Here's how the part is built. I have some questions about the finished solid (model axes, mm). A direction names the side the tool comes from. Give positions to 0.01 mm unless a question says otherwise; leave off trailing zeros. Loops run counter-clockwise (first coordinate to the right, second up) from the corner with the lowest first, then second, coordinate; pieces in that order, holes last. Notation, with made-up numbers: (44, -25) - (94, -25) arc R17 cw to (94, -7) - close; hole circle Ø5 at (67, -33.75). An arc over 180 degrees is marked (long way). Return JSON: item names as keys, results as strings. Group by question number.
(1) I need wall thicknesses on probe 1 along X at (y, z) = (10.25, 7.5) (3 decimals); probe 2 along Z at (x, y) = (19, 5.5) (3 decimals); probe 3 along X at (y, z) = (10.5, -8.5) (3 decimals). Which ranges of each line are inside material? Lowest first, please. Write a range as [from, to].
(2) If we section it at B-B (x = -4): Please give me the cut outline in (y, z) (3 decimals).
(3) If we section it at C-C (z = 5): Please give me the cut outline in (x, y) (3 decimals).
(4) On a 3-axis mill with a long thin cutter (end or side, diameter ignored), from which of +Z, -Z, +X, -X, +Y, -Y can I reach the whole of each face in a straight line? I mean faces 3 (the cylindrical face through (24.81, 14.64, -4.33)), 4 (the flat face through (22.5, -0.6, -8.985)), 5 (the flat face through (-23.6, -0.6, 8.985)). Say none if no direction works.
(5) For P1, Ø10, axis at x = -11, z = 5.5, coming from the +Y side; P2, Ø5, axis at x = -19, z = 4.5, coming from the -Y side; P3, Ø4, axis at x = 13.475, z = -11.175, coming from the -Y side; P4, Ø1.8, axis at x = -13.495, z = -11.175, coming from the +Y side, each with a flat end and sliding along its axis, tell me the tip position at first contact or that it passes through.
(6) If we mould it in two halves opening along X, with no side actions, what happens to faces 1 (the flat face through (12, -1.12, -11)), 2 (the cylindrical face through (-14.685, 2.007, -10.262))? For each: released by +X, released by -X, zero draft, split by the parting line, or undercut.
(7) If we section it at A-A (y = 3.25): Please give me the cut outline in (x, z) (3 decimals), then the cut area to 3 significant figures.
```python
from build123d import *

# Parameters (mm, degrees)
SKETCH_1_W          = 54.61
SKETCH_1_H          = 29.97
EXTRUDE_1_DEPTH     = 2.5
EXTRUDE_2_DEPTH     = 17
CUT_EXTRUDE_1_DEPTH = 30.97
SKETCH_4_R          = 1.145
CUT_EXTRUDE_2_DEPTH = 3.5
SKETCH_5_R          = 2.25
SKETCH_5_W          = 7.5
SKETCH_5_H          = 6
SKETCH_5_W_2        = 9.5
EXTRUDE_3_DEPTH     = 1.12
SKETCH_6_R          = 1.145
CUT_EXTRUDE_3_DEPTH = 4.62
SKETCH_7_R          = 1.5
CUT_EXTRUDE_4_DEPTH = 1
SKETCH_9_W          = 0.66
SKETCH_9_H          = 0.76
EXTRUDE_5_DEPTH     = 3
SKETCH_10_R         = 3.75
EXTRUDE_6_DEPTH     = 1
SKETCH_11_R         = 3
SKETCH_11_R_2       = 2
EXTRUDE_7_DEPTH     = 4
SKETCH_12_R         = 4.25
SKETCH_12_R_2       = 3.25
EXTRUDE_8_DEPTH     = 4
SKETCH5_W           = 26
SKETCH5_H           = 4
CUT_EXTRUDE4_DEPTH  = 17
BOSS_EXTRUDE1_DEPTH = 18
SKETCH7_W           = 2
SKETCH7_H           = 29.97
BOSS_EXTRUDE2_DEPTH = 1


with BuildPart() as part:
    # Эскиз1 → Бобышка-Вытянуть1 (new body)
    with BuildSketch(Plane(origin=(0, 0, 0), x_dir=(1, 0, 0), z_dir=(0, 1, 0))):
        Rectangle(SKETCH_1_W, SKETCH_1_H)
    extrude(amount=EXTRUDE_1_DEPTH)

    # Эскиз2 → Бобышка-Вытянуть2 (add)
    with BuildSketch(Plane(origin=(0, 2.5, 0), x_dir=(1, 0, 0), z_dir=(0, 1, 0))):
        with BuildLine():
            Line((27.305, -14.985), (-0.695, -14.985))
            Line((-0.695, -14.985), (-0.695, -13.485))
            Line((-0.695, -13.485), (23.305, -13.485))
            ThreePointArc((23.305, -13.485), (24.719213562, -12.899213562), (25.305, -11.485))
            Line((25.305, -11.485), (25.305, 11.485))
            ThreePointArc((25.305, 11.485), (24.719213562, 12.899213562), (23.305, 13.485))
            Line((23.305, 13.485), (-0.695, 13.485))
            Line((-0.695, 13.485), (-0.695, 14.985))
            Line((-0.695, 14.985), (27.305, 14.985))
            Line((27.305, 14.985), (27.305, -14.985))
        make_face()
    extrude(amount=EXTRUDE_2_DEPTH)

    # Эскиз3 → Вырез-Вытянуть1 (cut, through all)
    with BuildSketch(Plane.XY.offset(14.985)):
        Polygon((-0.695, 2.5), (25.305, 19.5), (-0.695, 19.5), align=None)
    extrude(amount=-CUT_EXTRUDE_1_DEPTH, mode=Mode.SUBTRACT)

    # Эскиз4 → Вырез-Вытянуть2 (cut, through all)
    with BuildSketch(Plane(origin=(0, 2.5, 0), x_dir=(1, 0, 0), z_dir=(0, 1, 0))):
        with Locations((-13.495, 11.175)):
            Circle(SKETCH_4_R)
        with Locations((-0.005, -11.175)):
            Circle(SKETCH_4_R)
        with Locations((13.475, 11.175)):
            Circle(SKETCH_4_R)
    extrude(amount=-CUT_EXTRUDE_2_DEPTH, mode=Mode.SUBTRACT)

    # Эскиз5 → Бобышка-Вытянуть3 (add)
    with BuildSketch(Plane.XZ):
        with Locations((-0.005, 11.175)):
            Circle(SKETCH_5_R)
        with Locations((13.475, -11.175)):
            Circle(SKETCH_5_R)
        with Locations((-13.495, -11.175)):
            Circle(SKETCH_5_R)
        with Locations((-23.555, 11.985)):
            Rectangle(SKETCH_5_W, SKETCH_5_H)
        with Locations((22.555, 11.985)):
            Rectangle(SKETCH_5_W_2, SKETCH_5_H)
        with Locations((22.555, -11.985)):
            Rectangle(SKETCH_5_W_2, SKETCH_5_H)
        with Locations((-23.555, -11.985)):
            Rectangle(SKETCH_5_W, SKETCH_5_H)
    extrude(amount=EXTRUDE_3_DEPTH)

    # Эскиз6 → Вырез-Вытянуть3 (cut, through all)
    with BuildSketch(Plane(origin=(0, 2.5, 0), x_dir=(1, 0, 0), z_dir=(0, 1, 0))):
        with Locations((-13.495, 11.175)):
            Circle(SKETCH_6_R)
        with Locations((13.475, 11.175)):
            Circle(SKETCH_6_R)
        with Locations((-0.005, -11.175)):
            Circle(SKETCH_6_R)
    extrude(amount=-CUT_EXTRUDE_3_DEPTH, mode=Mode.SUBTRACT)

    # Эскиз7 → Вырез-Вытянуть4 (cut)
    with BuildSketch(Plane(origin=(0, 2.5, 0), x_dir=(1, 0, 0), z_dir=(0, 1, 0))):
        with Locations((-13.495, 11.175)):
            Circle(SKETCH_7_R)
        with Locations((13.475, 11.175)):
            Circle(SKETCH_7_R)
        with Locations((-0.005, -11.175)):
            Circle(SKETCH_7_R)
    extrude(amount=-CUT_EXTRUDE_4_DEPTH, mode=Mode.SUBTRACT)

    # Эскиз9 → Бобышка-Вытянуть5 (add)
    with BuildSketch(Plane.XZ):
        with Locations((25.075, 6.35)):
            Rectangle(SKETCH_9_W, SKETCH_9_H)
        with Locations((25.075, -6.35)):
            Rectangle(SKETCH_9_W, SKETCH_9_H)
    extrude(amount=EXTRUDE_5_DEPTH)

    # Эскиз10 → Бобышка-Вытянуть6 (add)
    with BuildSketch(Plane.ZY.offset(-25.305)):
        with Locations((-6.35, 11.48)):
            Circle(SKETCH_10_R)
        with Locations((6.35, 11.48)):
            Circle(SKETCH_10_R)
    extrude(amount=EXTRUDE_6_DEPTH)

    # Эскиз11 → Бобышка-Вытянуть7 (add)
    with BuildSketch(Plane.ZY.offset(-24.305)):
        with Locations((-6.35, 11.48)):
            Circle(SKETCH_11_R)
        with Locations((-6.35, 11.48)):
            Circle(SKETCH_11_R_2, mode=Mode.SUBTRACT)
    extrude(amount=EXTRUDE_7_DEPTH)

    # Эскиз12 → Бобышка-Вытянуть8 (add)
    with BuildSketch(Plane.ZY.offset(-24.305)):
        with Locations((6.35, 11.48)):
            Circle(SKETCH_12_R)
        with Locations((6.35, 11.48)):
            Circle(SKETCH_12_R_2, mode=Mode.SUBTRACT)
    extrude(amount=EXTRUDE_8_DEPTH)

    # Sketch5 → Cut-Extrude4 (cut)
    with BuildSketch(Plane(origin=(0, 19.5, 0), x_dir=(1, 0, 0), z_dir=(0, 1, 0))):
        with Locations((12.305, -12.985)):
            Rectangle(SKETCH5_W, SKETCH5_H)
        with Locations((12.305, 12.985)):
            Rectangle(SKETCH5_W, SKETCH5_H)
    extrude(amount=-CUT_EXTRUDE4_DEPTH, mode=Mode.SUBTRACT)

    # Sketch6 → Boss-Extrude1 (add)
    with BuildSketch(Plane(origin=(0, 2.5, 0), x_dir=(1, 0, 0), z_dir=(0, 1, 0))):
        Polygon((25.305, 13.485), (25.305, 14.985), (-27.305, 14.985), (-27.305, -14.985), (25.305, -14.985), (25.305, -13.485), (-24.705, -13.485), (-24.705, 13.485), align=None)
    extrude(amount=BOSS_EXTRUDE1_DEPTH)

    # Sketch7 → Boss-Extrude2 (add)
    with BuildSketch(Plane(origin=(0, 19.5, 0), x_dir=(1, 0, 0), z_dir=(0, 1, 0))):
        with Locations((26.305, 0)):
            Rectangle(SKETCH7_W, SKETCH7_H)
    extrude(amount=BOSS_EXTRUDE2_DEPTH)


solid = part.part
```
Values:
{
 "1": {"probe 1": "[-27.305, -24.705], [24.305, 27.305]", "probe 2": "[-14.985, -13.485], [13.485, 14.985]", "probe 3": "[-27.305, -24.705], [20.305, 27.305]"},
 "2": {"outline": "(0, -14.985) - (20.5, -14.985) - (20.5, -13.485) - (2.5, -13.485) - (2.5, 13.485) - (20.5, 13.485) - (20.5, 14.985) - (0, 14.985) - close"},
 "3": {"outline": "(-27.305, 0) - (27.305, 0) - (27.305, 20.5) - (25.305, 20.5) - (25.305, 14.979) - (24.305, 14.979) - (24.305, 15.51) - (20.305, 15.51) - (20.305, 14.436) - (24.305, 14.436) - (24.305, 8.524) - (20.305, 8.524) - (20.305, 7.45) - (24.305, 7.45) - (24.305, 7.981) - (25.305, 7.981) - (25.305, 2.5) - (-24.705, 2.5) - (-24.705, 20.5) - (-27.305, 20.5) - close"},
 "4": {"face 3": "none", "face 4": "+X, -Y", "face 5": "-X, -Y"},
 "5": {"P1": "y = 2.5", "P2": "y = 0", "P3": "y = -1.12", "P4": "through"},
 "6": {"face 1": "zero draft", "face 2": "undercut"},
 "7": {"outline": "(-27.305, -14.985) - (27.305, -14.985) - (27.305, 14.985) - (-27.305, 14.985) - close; hole (-24.705, -13.485) - (25.305, -13.485) - (25.305, 13.485) - (-24.705, 13.485) - close", "area": "288 mm2"}
}
